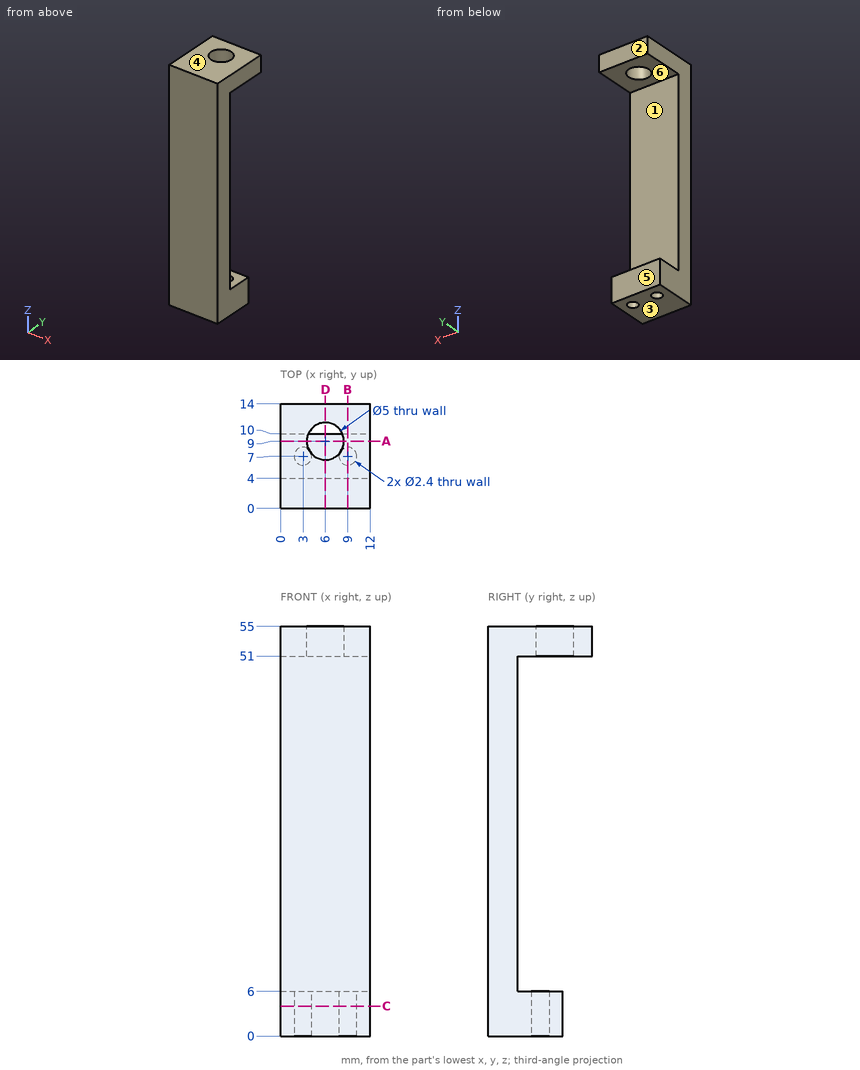
Input: dimensioned drawing with shaded views. Units: mm. Origin: part minimum x, y, z. A direction names the side the tool comes from. Round coordinates to 2 decimals unless told otherwise and drop trailing zeros. Loops run counter-clockwise (first coordinate to the right, second up) from the corner with the lowest first, then second, coordinate; pieces in that order, holes last. Notation, with made-up numbers: M -30.5,28.5 L -22.5,28.5 A21 cw -22.5,32.5 Z; hole C -9.75,-1.5 d10. An arc over 180 degrees is marked long. Answer in a Markdown table with one row per item. Add a question column.
1. Section B-B (x = 9). Output: boundary loops of the cut face in (y, z).
2. Section D-D (x = 6). Output: boundary loops of the cut face in (y, z), and give its area (3 significant figures).
3. Set-up query: the marked faces 4, 5 and 6. Return all of +Z, -Z, +X, -X, +Y, -Y with unobstructed straight access to the full face (end or side cutting, diameter ignored); none if empty.
4. Section C-C (z = 4). Output: boundary loops of the cut face in (x, y), and give its area (3 significant figures).
5. Mould query, pull axis Z, two halves, no side actions, for the marked faces 1, 2 and 3. Classes: released by +Z, released by -Z, zero draft, split by the parting line, or undercut.
6. Section A-A (y = 9). Output: boundary loops of the cut face in (x, z), and give its area (3 significant figures).
7. Contact query for flat-ended pins moving along their axis: pin 1 (6 mm diameter, centred on x = 8, z = 28, fed in from +Y); pin 2 (2 mm diameter, centred on x = 3, y = 7, fed in from -Z); pin 3 (1.8 mm diameter, centred on x = 9, z = 3, fed in from +Y). Output: stop coordinate, or through.
8. Ray query, probe 1 along Y at (x, z) = (3, 1.55); probe 2 along Z at (x, y) = (1.5, 9.75); probe 3 along Y at (x, z) = (3, 19). Return the intervals inside material, ascending.
Values follow:
| question | item | result |
|---|---|---|
| 1 | outline | M 0,0 L 5.8,0 L 5.8,6 L 4,6 L 4,51 L 14,51 L 14,55 L 0,55 Z; M 8.2,0 L 10,0 L 10,6 L 8.2,6 Z |
| 2 | outline | M 0,0 L 10,0 L 10,6 L 4,6 L 4,51 L 6.5,51 L 6.5,55 L 0,55 Z; M 11.5,51 L 14,51 L 14,55 L 11.5,55 Z |
| 2 | area | 276 mm^2 |
| 3 | face 4 | +Z, +X, -X, +Y, -Y |
| 3 | face 5 | -Z, +X, -X, +Y |
| 3 | face 6 | +X, -X, +Y |
| 4 | outline | M 0,0 L 12,0 L 12,10 L 0,10 Z; hole C 3,7 d2.4; hole C 9,7 d2.4 |
| 4 | area | 111 mm^2 |
| 5 | face 1 | undercut |
| 5 | face 2 | zero draft |
| 5 | face 3 | released by -Z |
| 6 | outline | M 0,0 L 12,0 L 12,6 L 0,6 Z; M 0,51 L 3.5,51 L 3.5,55 L 0,55 Z; M 8.5,51 L 12,51 L 12,55 L 8.5,55 Z |
| 6 | area | 100 mm^2 |
| 7 | pin 1 | y = 4 |
| 7 | pin 2 | z = 51 |
| 7 | pin 3 | y = 10 |
| 8 | probe 1 | 0 to 5.8, 8.2 to 10 |
| 8 | probe 2 | 0 to 6, 51 to 55 |
| 8 | probe 3 | 0 to 4 |
